from build123d import *

# Parameters (mm, degrees)
BOSS_EXTRUDE1_DEPTH     = 25.4
SKETCH2_R               = 4.191
CUT_EXTRUDE1_DEPTH      = 6.35
SKETCH3_W               = 50.8
SKETCH3_H               = 6.35
BOSS_EXTRUDE2_DEPTH     = 107.95
SKETCH5_W               = 31.75
SKETCH5_H               = 5
BOSS_EXTRUDE3_DEPTH     = 12.7
CUT_EXTRUDE2_DEPTH      = 143.062213484
CUT_EXTRUDE2_DEPTH_BACK = 143.062213484
SKETCH4_R               = 1.15


with BuildPart() as part:
    # Sketch1 → Boss-Extrude1 (new body)
    with BuildSketch(Plane.XY):
        with BuildLine():
            Line((-40.4, 0), (-15, 0))
            ThreePointArc((-15, 0), (-13.636673939, 6.248289676), (-9.794516817, 11.360785199))
            ThreePointArc((-9.794516817, 11.360785199), (-7.529268877, 13.921260066), (-6.02906924, 16.993194444))
            ThreePointArc((-6.02906924, 16.993194444), (0, 21.35), (6.02906924, 16.993194444))
            ThreePointArc((6.02906924, 16.993194444), (7.529268877, 13.921260066), (9.794516817, 11.360785199))
            ThreePointArc((9.794516817, 11.360785199), (13.636673939, 6.248289676), (15, 0))
            Line((15, 0), (40.4, 0))
            Line((40.4, 0), (40.4, 6.35))
            Line((40.4, 6.35), (21.298547486, 6.35))
            ThreePointArc((21.298547486, 6.35), (19.237888282, 11.128983757), (16.122349869, 15.297727273))
            ThreePointArc((16.122349869, 15.297727273), (13.714805021, 18.915005141), (12.667560611, 23.132142857))
            ThreePointArc((12.667560611, 23.132142857), (0, 34.925), (-12.667560611, 23.132142857))
            ThreePointArc((-12.667560611, 23.132142857), (-13.714805021, 18.915005141), (-16.122349869, 15.297727273))
            ThreePointArc((-16.122349869, 15.297727273), (-19.237888282, 11.128983757), (-21.298547486, 6.35))
            Line((-21.298547486, 6.35), (-40.4, 6.35))
            Line((-40.4, 6.35), (-40.4, 0))
        make_face()
    boss_extrude1 = extrude(amount=BOSS_EXTRUDE1_DEPTH)

    # Sketch2 → Cut-Extrude1 (cut)
    with BuildSketch(Plane(origin=(0, 6.35, 0), x_dir=(1, 0, 0), z_dir=(0, 1, 0))):
        with Locations(Location((-30.798547486, -12.7, 0), (0, 0, 180))):
            Circle(SKETCH2_R)
        with Locations(Location((30.798553886, -12.7, 0), (0, 0, 180))):
            Circle(SKETCH2_R)
    cut_extrude1 = extrude(amount=-CUT_EXTRUDE1_DEPTH, mode=Mode.SUBTRACT)

    # Sketch3 → Boss-Extrude2 (add)
    with BuildSketch(Plane(origin=(0, 0, 0), x_dir=(-1, 0, 0), z_dir=(0, 0, -1))):
        with Locations((0, 24.525)):
            Rectangle(SKETCH3_W, SKETCH3_H)
    extrude(amount=BOSS_EXTRUDE2_DEPTH)

    # Mirror1: Boss-Extrude1, Cut-Extrude1 across plane
    add(boss_extrude1.mirror(Plane(origin=(0, 0, -53.975), x_dir=(1, 0, 0), z_dir=(0, 0, -1))))
    add(cut_extrude1.mirror(Plane(origin=(0, 0, -53.975), x_dir=(1, 0, 0), z_dir=(0, 0, -1))), mode=Mode.SUBTRACT)

    # Sketch5 → Boss-Extrude3 (add)
    with BuildSketch(Plane(origin=(0, 27.7, 0), x_dir=(1, 0, 0), z_dir=(0, 1, 0))):
        with Locations((0, 6.31)):
            Rectangle(SKETCH5_W, SKETCH5_H)
        with Locations((0, 101.3899878)):
            Rectangle(SKETCH5_W, SKETCH5_H)
    extrude(amount=BOSS_EXTRUDE3_DEPTH)

    # Sketch4 → Cut-Extrude2 (cut, two sides: drawn at the far end of the back side and taken through both)
    with BuildSketch(Plane(origin=(0, 27.7, 0), x_dir=(1, 0, 0), z_dir=(0, 1, 0)).offset(-CUT_EXTRUDE2_DEPTH_BACK)):
        with Locations(Location((9.4, 101.349999992, 0), (0, 0, 180))):
            Circle(SKETCH4_R)
        with Locations(Location((-8.6, 101.35, 0), (0, 0, 180))):
            Circle(SKETCH4_R)
        with Locations(Location((9.4, 6.35, 0), (0, 0, 180))):
            Circle(SKETCH4_R)
        with Locations(Location((-8.6, 6.35, 0), (0, 0, 180))):
            Circle(SKETCH4_R)
    extrude(amount=CUT_EXTRUDE2_DEPTH + CUT_EXTRUDE2_DEPTH_BACK, mode=Mode.SUBTRACT)


solid = part.part
Check sheet for the modelled part. Datum: model origin and axes. Units: mm. A direction names the side the tool comes from. Round coordinates to 2 decimals unless told otherwise and drop trailing zeros. Write each loop counter-clockwise with the first axis right and the second up, starting at its lowest first coordinate (ties: lowest second). Pieces come first, ordered by that corner, then holes. Notation, with made-up numbers: (73.25, 31.5) - (127.25, 31.5) arc R29 ccw to (127.25, 52.5) - close; hole circle Ø5 at (47, -11.75). An arc over 180 degrees is marked (long way). Return JSON: item names as keys, results as strings.
Q1. Scan lines: L1, parallel to Z at x = 9.4, y = 31; L2, parallel to Z at x = 9.4, y = 26.75; L3, parallel to Z at x = 5.5, y = 28. Record each from-to range of solid material in increasing order. Write a range as from..to.
Returned:
{"L1": "z = -103.89..-102.5, -100.2..-98.89, -8.81..-7.5, -5.2..-3.81", "L2": "z = -133.35..-102.5, -100.2..-7.5, -5.2..25.4", "L3": "z = -133.35..-107.95, -103.89..-98.89, -8.81..-3.81, 0..25.4"}
Q2. Depth check by flat-ended pin: P1, Ø15.5, axis at x = 27.5, z = 9.5, coming from the +Y side; P2, Ø7, axis at x = 21, y = 24.5, coming from the +Z side; P3, Ø3, axis at x = 10.5, y = 6.5, coming from the -Z side; P4, Ø3, axis at x = -8.6, z = -101.35, coming from the -Y side. Enter the tip coordinate at first touch or a pass-through.
Returned:
{"P1": "stops at y = 10.19", "P2": "stops at z = 0", "P3": "passes through", "P4": "stops at y = 21.35"}
Q3. Cross-section at A-A (z = -120.65). Record the boundary of the cut face in (x, y) (3 decimals).
Returned:
{"outline": "(-40.4, 0) - (-34.99, 0) - (-34.99, 6.35) - (-40.4, 6.35) - close; (-26.608, 0) - (-15, 0) arc R15 cw to (-9.795, 11.361) arc R12.7 ccw to (-6.029, 16.993) arc R6.35 cw to (6.029, 16.993) arc R12.7 ccw to (9.795, 11.361) arc R15 cw to (15, 0) - (26.608, 0) - (26.608, 6.35) - (21.299, 6.35) arc R22.225 ccw to (16.122, 15.298) arc R12.7 cw to (12.668, 23.132) arc R12.7 ccw to (-12.668, 23.132) arc R12.7 cw to (-16.122, 15.298) arc R22.225 ccw to (-21.299, 6.35) - (-26.608, 6.35) - close; (34.99, 0) - (40.4, 0) - (40.4, 6.35) - (34.99, 6.35) - close"}
Q4. Cross-section at B-B (y = 30). Record the boundary of the cut face in (x, z) (3 decimals), then the cut area to 3 significant figures.
Returned:
{"outline": "(-15.875, -103.89) - (15.875, -103.89) - (15.875, -98.89) - (-15.875, -98.89) - close; (-15.875, -8.81) - (15.875, -8.81) - (15.875, -3.81) - (-15.875, -3.81) - close; (-10.042, -133.35) - (10.042, -133.35) - (10.042, -107.95) - (-10.042, -107.95) - close; (-10.042, 0) - (10.042, 0) - (10.042, 25.4) - (-10.042, 25.4) - close; hole circle Ø2.3 at (-8.6, -101.35); hole circle Ø2.3 at (-8.6, -6.35); hole circle Ø2.3 at (9.4, -101.35); hole circle Ø2.3 at (9.4, -6.35)", "area": "1,320 mm²"}
Q5. Cross-section at C-C (z = -16.5). Record the boundary of the cut face in (x, y).
Returned:
{"outline": "(-25.4, 21.35) - (25.4, 21.35) - (25.4, 27.7) - (-25.4, 27.7) - close"}
Q6. Access from +Z, -Z, +X, -X, +Y, -Y to the whole of each face (thin tool, end or side, straight path). Record for faces 1 (the flat face through (19, 25, -107.95)), 2 (the flat face through (0, 21.35, -53)), 3 (the cylindrical face through (13.6, 6.33, -120.47)).
Returned:
{"face 1": "-Z, +X, +Y", "face 2": "+X, -X, -Y", "face 3": "+Z, -Z, -Y"}
